```python
from build123d import *

# Parameters (mm, degrees)
F0_W     = 61.25
F0_H     = 61.25
F1_DEPTH = 10
F3_DEPTH = 80
F4_R     = 1
F4_R_2   = 1.25
F5_DEPTH = 80


with BuildPart() as f1:
    # F0 (on Front) → F1 (new body)
    with BuildSketch(Plane.XZ):
        with Locations((30.625, 30.625)):
            Rectangle(F0_W, F0_H)
    extrude(amount=F1_DEPTH)

    # F2 (on face) → F3 (cut)
    with BuildSketch(Plane.YZ.offset(61.25)):
        with BuildLine():
            Line((-10, 56.25), (-10, 5))
            Line((-10, 5), (-8.5, 5))
            ThreePointArc((-8.5, 5), (-4.964466, 6.464466), (-3.5, 10))
            Line((-3.5, 10), (-3.5, 51.25))
            ThreePointArc((-3.5, 51.25), (-4.964466, 54.785534), (-8.5, 56.25))
            Line((-8.5, 56.25), (-10, 56.25))
        make_face()
    extrude(amount=-F3_DEPTH, mode=Mode.SUBTRACT)

    # F4 (on face) → F5 (cut)
    with BuildSketch(Plane(origin=(0, 0, 0), x_dir=(1, 0, 0), z_dir=(0, 0, -1))):
        with Locations((56.25, 7)):
            Circle(F4_R)
        with Locations((5, 7)):
            Circle(F4_R_2)
    extrude(amount=-F5_DEPTH, mode=Mode.SUBTRACT)


solid = f1.part
```
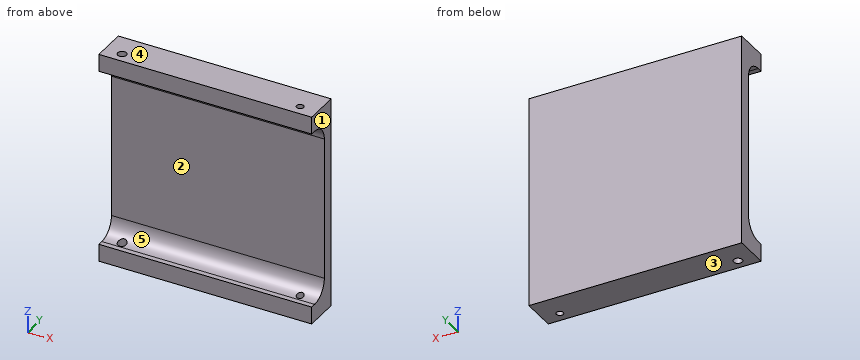
Build history of the part. All positions in model axes, mm. Face numbers are marked on the shaded views. A direction names the side the tool comes from. Round coordinates to 2 decimals unless told otherwise and drop trailing zeros. Write each loop counter-clockwise with the first axis right and the second up, starting at its lowest first coordinate (ties: lowest second). Pieces come first, ordered by that corner, then holes. Notation, with made-up numbers: (57, 18) -> (113, 18) arc R10 ccw to (113, 35) -> close; hole circle Ø1 at (38, 26). An arc over 180 degrees is marked (long way). Put each result on its own line as item: value.
Item 1: Slice it at D-D, the plane x = 5. Give the cut face in (y, z).
Here are the results:
outline: (-10, 0) -> (-8.25, 0) -> (-8.25, 5.01) arc R5 cw to (-8.5, 5) -> (-10, 5) -> close; (-10, 56.25) -> (-8.5, 56.25) arc R5 cw to (-8.25, 56.24) -> (-8.25, 61.25) -> (-10, 61.25) -> close; (-5.75, 0) -> (0, 0) -> (0, 61.25) -> (-5.75, 61.25) -> (-5.75, 55.43) arc R5 cw to (-3.5, 51.25) -> (-3.5, 10) arc R5 cw to (-5.75, 5.82) -> close
Item 2: Slice it at A-A, the plane y = -7. Give the cut face in (x, z), plus the area to 3 significant figures.
Here are the results:
outline: (0, 0) -> (3.75, 0) -> (3.75, 5.23) -> (0, 5.23) -> close; (0, 56.02) -> (3.75, 56.02) -> (3.75, 61.25) -> (0, 61.25) -> close; (6.25, 0) -> (55.25, 0) -> (55.25, 5.23) -> (6.25, 5.23) -> close; (6.25, 56.02) -> (55.25, 56.02) -> (55.25, 61.25) -> (6.25, 61.25) -> close; (57.25, 0) -> (61.25, 0) -> (61.25, 5.23) -> (57.25, 5.23) -> close; (57.25, 56.02) -> (61.25, 56.02) -> (61.25, 61.25) -> (57.25, 61.25) -> close
area: 594 mm^2
Item 3: Two-plate mould, pull along Z, no slides. Class the marked faces 3, 4 and 5: pulls with the +Z half, pulls with the -Z half, needs draft (parallel to the pull), parting line crosses it, or undercut.
Here are the results:
face 3: pulls with the -Z half
face 4: pulls with the +Z half
face 5: undercut
Item 4: Slice it at C-C, the plane z = 37. Give the cut face in (x, y), plus the area to 3 significant figures.
Here are the results:
outline: (0, -3.5) -> (61.25, -3.5) -> (61.25, 0) -> (0, 0) -> close
area: 214 mm^2
Item 5: Flat gauge pins, fed straight in: P1, Ø2.5, axis at x = 56.25, y = -7, coming from the -Z side; P2, Ø12.5, axis at x = 41.5, z = 29, coming from the -Y side. Where does each tip first touch, or does it go through?
Here are the results:
P1: stops at z = 0
P2: stops at y = -3.5
Item 6: Tool access for the marked faces 1 and 2: list every direction of +Z, -Z, +X, -X, +Y, -Y with a clear straight run to the whole face (end or side of a thin tool).
Here are the results:
face 1: +Z, -Z, +X, +Y, -Y
face 2: +X, -X, -Y
Item 7: Slice it at B-B, the plane x = 56.25. Give the cut face in (y, z), plus the area to 3 significant figures.
Here are the results:
outline: (-10, 0) -> (-8, 0) -> (-8, 5.03) arc R5 cw to (-8.5, 5) -> (-10, 5) -> close; (-10, 56.25) -> (-8.5, 56.25) arc R5 cw to (-8, 56.22) -> (-8, 61.25) -> (-10, 61.25) -> close; (-6, 0) -> (0, 0) -> (0, 61.25) -> (-6, 61.25) -> (-6, 55.58) arc R5 cw to (-3.5, 51.25) -> (-3.5, 10) arc R5 cw to (-6, 5.67) -> close
area: 269 mm^2
Item 8: Wall check: probe 1 along X at (y, z) = (-7, 58.15); probe 2 along Y at (x, z) = (5, 58.3); probe 3 along Z at (x, y) = (39, -9). Give the ranges that are in metal, low to high. Write a range as from..to.
Here are the results:
probe 1: x = 0..3.75, 6.25..55.25, 57.25..61.25
probe 2: y = -10..-8.25, -5.75..0
probe 3: z = 0..5, 56.25..61.25
